Source: CAD feature listing. Evaluate the final solid. Frame: model axes, mm. Face numbers are marked on the shaded views. A direction names the side the tool comes from. Round coordinates to 2 decimals unless told otherwise and drop trailing zeros. Loops run counter-clockwise (first coordinate to the right, second up) from the corner with the lowest first, then second, coordinate; pieces in that order, holes last. Notation, with made-up numbers: (61.25, 63.5) -> (100.25, 63.5) arc R11 ccw to (100.25, 68.5) -> close; hole circle Ø4 at (4.25, 75). An arc over 180 degrees is marked (long way). Put each result on its own line as item: value. Start each with the question number.
1. Cut plane C-C (y = -571.5). Return the cut outline in (x, z).
2. Contact query for flat-ended pins moving along their axis: pin 1 (2 mm diameter, centred on x = 1006, y = -221.5, fed in from +Z); pin 2 (2 mm diameter, centred on y = -1089.5, z = 693.5, fed in from +X). Output: stop coordinate, or through.
3. Set-up query: the marked faces 1, 2 and 3. Return all of +Z, -Z, +X, -X, +Y, -Y with unobstructed straight access to the full face (end or side cutting, diameter ignored); none if empty.
4. Cut plane D-D (x = 1300). Return the cut outline in (y, z).
5. Material intervals for L1, parallel to Y at x = 835, z = 983.5; L2, parallel to X at y = -1402.5, z = 675.5; L3, parallel to Z at x = 1182.5, y = -655.5, sorted ascending.
6. Cut plane A-A (x = 746.5). Return the cut outline in (y, z).
7. Cut plane B-B (z = 909). Return the cut outline in (x, y).
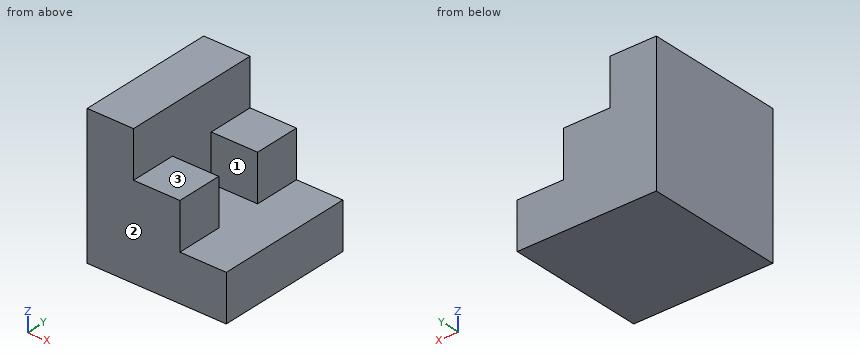
```python
from build123d import *

# Parameters (mm, degrees)
F0_W     = 1524
F0_H     = 1524
F1_DEPTH = 1524
F3_DEPTH = 1524
F4_W     = 508
F4_H     = 508
F5_DEPTH = 508


with BuildPart() as f1:
    # F0 (on Front) → F1 (new body)
    with BuildSketch(Plane.XZ):
        with Locations((762, 762)):
            Rectangle(F0_W, F0_H)
    extrude(amount=F1_DEPTH)

    # F2 (on face) → F3 (cut)
    with BuildSketch(Plane.XZ.offset(1524)):
        Polygon((1524, 1524), (508, 1524), (508, 1016), (1016, 1016), (1016, 508), (1524, 508), align=None)
    extrude(amount=-F3_DEPTH, mode=Mode.SUBTRACT)

    # F4 (on face) → F5 (cut)
    with BuildSketch(Plane.YZ.offset(1016)):
        with Locations((-762, 762)):
            Rectangle(F4_W, F4_H)
    extrude(amount=-F5_DEPTH, mode=Mode.SUBTRACT)


solid = f1.part
```
Solution:
1. outline: (0, 0) -> (1524, 0) -> (1524, 508) -> (508, 508) -> (508, 1524) -> (0, 1524) -> close
2. pin 1: stops at z = 1016
2. pin 2: stops at x = 1016
3. face 1: +Z, +X
3. face 2: +Z, -Z, +X, -X, -Y
3. face 3: +Z, +X, +Y, -Y
4. outline: (-1524, 0) -> (0, 0) -> (0, 508) -> (-1524, 508) -> close
5. L1: y = -1524 to -1016, -508 to 0
5. L2: x = 0 to 1016
5. L3: z = 0 to 508
6. outline: (-1524, 0) -> (0, 0) -> (0, 1016) -> (-508, 1016) -> (-508, 508) -> (-1016, 508) -> (-1016, 1016) -> (-1524, 1016) -> close
7. outline: (0, -1524) -> (1016, -1524) -> (1016, -1016) -> (508, -1016) -> (508, -508) -> (1016, -508) -> (1016, 0) -> (0, 0) -> close
